from build123d import *

# Parameters (mm, degrees)
SKETCH5_W           = 215
SKETCH5_H           = 30
BOSS_EXTRUDE3_DEPTH = 50
CUT_EXTRUDE2_DEPTH  = 123.295748086
CUT_EXTRUDE3_DEPTH  = 123.295748086
SKETCH8_W           = 8
SKETCH8_H           = 30
BOSS_EXTRUDE4_DEPTH = 25
SKETCH9_W           = 7
SKETCH9_H           = 5
BOSS_EXTRUDE5_DEPTH = 7
CUT_EXTRUDE4_DEPTH  = 135.466538589
SKETCH11_R          = 2
CUT_EXTRUDE5_DEPTH  = 221.678499179
SKETCH12_R          = 3.740099061
SKETCH12_R_2        = 4.034215751
CUT_EXTRUDE6_DEPTH  = 134.295377202


with BuildPart() as part:
    # Sketch5 → Boss-Extrude3 (new body)
    with BuildSketch(Plane.XY):
        Rectangle(SKETCH5_W, SKETCH5_H)
    extrude(amount=BOSS_EXTRUDE3_DEPTH)

    # Sketch6 → Cut-Extrude2 (cut, through all)
    with BuildSketch(Plane(origin=(0, 15, 0), x_dir=(1, 0, 0), z_dir=(0, 1, 0))):
        Polygon((-107.5, -32.077014326), (-52.338722055, -50), (-107.5, -50), align=None)
    extrude(amount=-CUT_EXTRUDE2_DEPTH, mode=Mode.SUBTRACT)

    # Sketch7 → Cut-Extrude3 (cut, through all)
    with BuildSketch(Plane(origin=(0, 15, 0), x_dir=(1, 0, 0), z_dir=(0, 1, 0))):
        Polygon((107.5, -42), (-51.071646532, -42), (-107.5, -23.665316532), (-107.5, 0), (107.5, 0), align=None)
    extrude(amount=-CUT_EXTRUDE3_DEPTH, mode=Mode.SUBTRACT)

    # Sketch8 → Boss-Extrude4 (add)
    with BuildSketch(Plane.XY.offset(50)):
        with Locations((103.5, 0)):
            Rectangle(SKETCH8_W, SKETCH8_H)
    extrude(amount=BOSS_EXTRUDE4_DEPTH)

    # Sketch9 → Boss-Extrude5 (add)
    with BuildSketch(Plane.ZY.offset(-99.5)):
        with Locations((53.5, -12.5)):
            Rectangle(SKETCH9_W, SKETCH9_H)
        with Locations((53.5, 12.5)):
            Rectangle(SKETCH9_W, SKETCH9_H)
    extrude(amount=BOSS_EXTRUDE5_DEPTH)

    # Sketch10 → Cut-Extrude4 (cut, through all)
    with BuildSketch(Plane.XZ.offset(15)):
        Polygon((92.5, 50), (99.5, 57), (92.5, 57), align=None)
    extrude(amount=-CUT_EXTRUDE4_DEPTH, mode=Mode.SUBTRACT)

    # Sketch11 → Cut-Extrude5 (cut, through all)
    with BuildSketch(Plane.ZY.offset(-99.5)):
        with Locations(Location((62.5, 0, 0), (0, 0, 270))):
            Circle(SKETCH11_R)
    extrude(amount=-CUT_EXTRUDE5_DEPTH, mode=Mode.SUBTRACT)

    # Sketch12 → Cut-Extrude6 (cut, through all)
    with BuildSketch(Plane(origin=(-19.692534532, 0, 60.607389333), x_dir=(0.9510565162951554, 0, 0.3090169943749418), z_dir=(-0.3090169943749418, 0, 0.9510565162951554))):
        with Locations((-77.326232946, 7.5)):
            Circle(SKETCH12_R)
        with Locations((-77.326232946, -7.5)):
            Circle(SKETCH12_R_2)
    extrude(amount=-CUT_EXTRUDE6_DEPTH, mode=Mode.SUBTRACT)


solid = part.part
Work out the finished part from the listing and answer in its coordinate system (mm). A direction names the side the tool comes from. Coordinates: 2 decimals unless noted, no trailing zeros. Write each loop counter-clockwise with the first axis right and the second up, starting at its lowest first coordinate (ties: lowest second). Pieces come first, ordered by that corner, then holes. Notation, with made-up numbers: M -27,51 L 26,51 A23 cw 26,90 Z; hole C 86.25,4.5 d3. An arc over 180 degrees is marked long. Write item = value, one per line.
1. The part is cut by section A-A (y = 0). Determine the outline of the cut face in (x, z), then the cut area to 3 significant figures.
Solution:
outline = M -107.5,23.67 L -51.07,42 L 107.5,42 L 107.5,60.5 L 99.5,60.5 L 99.5,50 L -52.34,50 L -107.5,32.08 Z; M 99.5,64.5 L 107.5,64.5 L 107.5,75 L 99.5,75 Z
area = 1,910 mm2
2. The part is cut by section C-C (z = 52). Determine the outline of the cut face in (x, y).
Solution:
outline = M 94.5,-15 L 107.5,-15 L 107.5,15 L 94.5,15 L 94.5,10 L 99.5,10 L 99.5,-10 L 94.5,-10 Z
3. Determine the mould class of faces 4 (the face through (103, 0, 75)), 5 (the face through (96, -12.5, 53.5)), 6 (the face through (-88.73, 6.07, 34.03)), 7 (the face through (-88.356, -6.288, 34.15)) for opening direction X: released by +X, released by -X, zero draft, split by the parting line, or undercut.
Solution:
face_4 = zero draft
face_5 = released by -X
face_6 = undercut
face_7 = undercut
4. For faces 1 (the face through (29, 0, 42)), 2 (the face through (107.5, 0, 58)), 3 (the face through (97, -10, 53)), determine the directions among +Z, -Z, +X, -X, +Y, -Y from which every point of the face is accessible in a straight line to the end or side of a thin tool.
Solution:
face_1 = -Z, +X, +Y, -Y
face_2 = +Z, -Z, +X, +Y, -Y
face_3 = +Z, -X
5. Flat-ended cylindrical pins translate along their axes: pin 1 (10 mm diameter, centred on y = -5.5, z = 42, fed in from -X); pin 2 (15 mm diameter, centred on x = 61, y = 3.5, fed in from -Z); pin 3 (15 mm diameter, centred on x = 34, y = -4.5, fed in from +Z). Find the tip coordinate at first contact, or state that the pin passes through.
Solution:
pin_1 = -91.53
pin_2 = 42
pin_3 = 50
6. The part is cut by section B-B (z = 62.5). Determine the outline of the cut face in (x, y), then the cut area to 3 significant figures.
Solution:
outline = M 99.5,-15 L 107.5,-15 L 107.5,-2 L 99.5,-2 Z; M 99.5,2 L 107.5,2 L 107.5,15 L 99.5,15 Z
area = 208 mm2
7. Straight lines are drawn through the part: line 1 (Z direction, x = 104, y = 0); line 2 (X direction, y = -12, z = 72); line 3 (Z direction, x = 18, y = -6.5). For each, find the intervals that lie inside material, in ascending order. Write a range as from..to.
Solution:
line_1 = 42..60.5, 64.5..75
line_2 = 99.5..107.5
line_3 = 42..50
8. The part is cut by section D-D (x = 87.5). Determine the outline of the cut face in (y, z).
Solution:
outline = M -15,42 L 15,42 L 15,50 L -15,50 Z
